The listing builds one solid part. Answer for the finished solid, in the listing's coordinates (mm). A direction names the side the tool comes from. Give positions to 0.01 mm unless a question says otherwise; leave off trailing zeros. Order: outer loops, then holes, each group sorted by start corner. A loop starts at its lowest first (then second) coordinate and runs counter-clockwise, first axis right, second up. Notation, with made-up numbers: (-2.75, -8) - (37.25, -8) arc R15 ccw to (37.25, -3) - close; hole circle Ø11 at (-27, 8.25). An arc over 180 degrees is marked (long way). Answer in a Markdown table with one row per item.
from build123d import *

# Parameters (mm, degrees)
F0_W     = 69.85
F0_H     = 31.75
F1_DEPTH = 38.1
F3_DEPTH = 12.7
F5_DEPTH = 12.7
F7_DEPTH = 25.401


# Not quite as in the source:
# - a feature names something its author has since deleted; it is built from what else it names


with BuildPart() as f1:
    # F0 (on Front) → F1 (new body)
    with BuildSketch(Plane.XZ):
        with Locations((-34.925, 15.875)):
            Rectangle(F0_W, F0_H)
    extrude(amount=F1_DEPTH)

    # F2 (on face) → F3 (cut)
    with BuildSketch(Plane(origin=(0, 0, 0), x_dir=(-1, 0, 0), z_dir=(0, 1, 0))):
        Polygon((69.85, 31.75), (19.05, 31.75), (31.75, 0), (69.85, 0), align=None)
    extrude(amount=-F3_DEPTH, mode=Mode.SUBTRACT)

    # F4 (on face) → F5 (cut)
    with BuildSketch(Plane.XZ.offset(38.1)):
        Polygon((-31.75, 0), (-19.05, 31.75), (-69.85, 31.75), (-69.85, 0), align=None)
    extrude(amount=-F5_DEPTH, mode=Mode.SUBTRACT)

    # F6 (on face) → F7 (cut, through all)
    with BuildSketch(Plane.XZ.offset(25.4)):
        Polygon((-69.85, 0), (-50.8, 31.75), (-69.85, 31.75), align=None)
    extrude(amount=-F7_DEPTH, mode=Mode.SUBTRACT)


solid = f1.part
Item 1: Find section D-D on x = -44. Write down the section's boundary in (y, z).
Answer block:
| item | result |
|---|---|
| outline | (-25.4, 0) - (-12.7, 0) - (-12.7, 31.75) - (-25.4, 31.75) - close |
Item 2: Find section B-B on y = -33.5. Write down the section's boundary in (x, z).
Answer block:
| item | result |
|---|---|
| outline | (-31.75, 0) - (0, 0) - (0, 31.75) - (-19.05, 31.75) - close |
Item 3: Find section C-C on x = -21. Write down the section's boundary in (y, z) (3 decimals).
Answer block:
| item | result |
|---|---|
| outline | (-38.1, 0) - (0, 0) - (0, 26.875) - (-12.7, 26.875) - (-12.7, 31.75) - (-25.4, 31.75) - (-25.4, 26.875) - (-38.1, 26.875) - close |
Item 4: Find section A-A on z = 6.5. Write down the section's boundary in (x, y), then the cut area to 3 significant figures.
Answer block:
| item | result |
|---|---|
| outline | (-65.95, -25.4) - (-29.15, -25.4) - (-29.15, -38.1) - (0, -38.1) - (0, 0) - (-29.15, 0) - (-29.15, -12.7) - (-65.95, -12.7) - close |
| area | 1,580 mm² |
Item 5: Which of the six approach directions +Z, -Z, +X, -X, +Y, -Y give full straight-line access (tool end or side, diameter ignored) to faces 1 (the face through (-45, -25.4, 16)), 2 (the face through (-25.31, -6.26, 16.1)), 3 (the face through (-13, 0, 16))?
Answer block:
| item | result |
|---|---|
| face 1 | +Z, -X, -Y |
| face 2 | +Z, -X, +Y |
| face 3 | +Z, -Z, +X, -X, +Y |
Item 6: Consider line 1 (Z direction, x = -66, y = -24.5); line 2 (X direction, y = -19, z = 6); line 3 (X direction, y = -1.5, z = 28.5). Determine where each line is inside the solid, lowest interval first.
Answer block:
| item | result |
|---|---|
| line 1 | 0 to 6.42 |
| line 2 | -66.25 to 0 |
| line 3 | -20.35 to 0 |
Item 7: Each of these flat-tipped pins is pushed along its axis until it touches: P1, Ø3, axis at y = -24, z = 3.5, coming from the -X side; P2, Ø4, axis at x = -37, y = -26.5, coming from the +Z side; P3, Ø10, axis at x = -56.5, z = 18, coming from the +Y side; P4, Ø2, axis at x = -27, z = 16, coming from the -Y side. Where does it stop, or does it pass through?
Answer block:
| item | result |
|---|---|
| P1 | x = -68.65 |
| P2 | z = 31.75 |
| P3 | y = -12.7 |
| P4 | y = -25.4 |
